```python
from build123d import *

# Parameters (mm, degrees)
SKIZZE1_W                        = 199
SKIZZE1_H                        = 420
AUFSATZ_LINEAR_AUSTRAGEN1_DEPTH  = 10
SKIZZE5_W                        = 199
SKIZZE5_H                        = 85
SCHNITT_LINEAR_AUSTRAGEN2_DEPTH  = 10
SKIZZE20_R                       = 1.7
SCHNITT_LINEAR_AUSTRAGEN12_DEPTH = 233.594604409
SKIZZE21_W                       = 134.422077922
SKIZZE21_H                       = 75
SCHNITT_LINEAR_AUSTRAGEN13_DEPTH = 233.594604409
SCHNITT_LINEAR_AUSTRAGEN14_DEPTH = 233.594604409
AUFSATZ_LINEAR_AUSTRAGEN6_DEPTH  = 10
SKIZZE25_R                       = 1.7
SCHNITT_LINEAR_AUSTRAGEN15_DEPTH = 233.594604409
SCHNITT_LINEAR_AUSTRAGEN16_DEPTH = 290.484023739
VERRUNDUNG1_R                    = 3
SKIZZE27_R                       = 1.7
SCHNITT_LINEAR_AUSTRAGEN17_DEPTH = 233.594604409
SCHNITT_LINEAR_AUSTRAGEN18_DEPTH = 5


with BuildPart() as part:
    # Skizze1 → Aufsatz-Linear austragen1 (new body)
    with BuildSketch(Plane(origin=(0, 0, 0), x_dir=(1, 0, 0), z_dir=(0, 1, 0))):
        Rectangle(SKIZZE1_W, SKIZZE1_H)
    extrude(amount=AUFSATZ_LINEAR_AUSTRAGEN1_DEPTH)

    # Skizze5 → Schnitt-Linear austragen2 (cut)
    with BuildSketch(Plane(origin=(0, 10, 0), x_dir=(1, 0, 0), z_dir=(0, 1, 0))):
        Polygon((99.5, -210), (18, -210), (99.5, -56), align=None)
        Polygon((-18, -210), (-99.5, -56), (-99.5, -210), align=None)
        with Locations((0, 167.5)):
            Rectangle(SKIZZE5_W, SKIZZE5_H)
        Polygon((67.211038961, -56), (-67.211038961, -56), (-2.646103896, -178), (2.646103896, -178), align=None)
    extrude(amount=-SCHNITT_LINEAR_AUSTRAGEN2_DEPTH, mode=Mode.SUBTRACT)

    # Skizze20 → Schnitt-Linear austragen12 (cut, through all)
    with BuildSketch(Plane(origin=(0, 10, 0), x_dir=(1, 0, 0), z_dir=(0, 1, 0))):
        with Locations(Location((90.5, 119.52, 0), (0, 0, 270))):
            Circle(SKIZZE20_R)
        with Locations(Location((48.5, 119.52, 0), (0, 0, 270))):
            Circle(SKIZZE20_R)
        with Locations(Location((-48.5, 119.52, 0), (0, 0, 90))):
            Circle(SKIZZE20_R)
        with Locations(Location((-90.5, 119.52, 0), (0, 0, 90))):
            Circle(SKIZZE20_R)
        with Locations(Location((87, 43.82, 0), (0, 0, 270))):
            Circle(SKIZZE20_R)
        with Locations(Location((52, 43.82, 0), (0, 0, 270))):
            Circle(SKIZZE20_R)
        with Locations(Location((-87, 43.82, 0), (0, 0, 90))):
            Circle(SKIZZE20_R)
        with Locations(Location((-52, 43.82, 0), (0, 0, 90))):
            Circle(SKIZZE20_R)
    extrude(amount=-SCHNITT_LINEAR_AUSTRAGEN12_DEPTH, mode=Mode.SUBTRACT)

    # Skizze21 → Schnitt-Linear austragen13 (cut, through all)
    with BuildSketch(Plane(origin=(0, 10, 0), x_dir=(1, 0, 0), z_dir=(0, 1, 0))):
        with Locations((0, -18.5)):
            Rectangle(SKIZZE21_W, SKIZZE21_H)
    extrude(amount=-SCHNITT_LINEAR_AUSTRAGEN13_DEPTH, mode=Mode.SUBTRACT)

    # Skizze22 → Schnitt-Linear austragen14 (cut, through all)
    with BuildSketch(Plane(origin=(0, 10, 0), x_dir=(1, 0, 0), z_dir=(0, 1, 0))):
        with BuildLine():
            Line((-67.211038961, -56), (-2.646103896, -178))
            ThreePointArc((-2.646103896, -178), (-52.825886854, -126.471631215), (-67.211038961, -56))
        make_face()
    schnitt_linear_austragen14 = extrude(amount=-SCHNITT_LINEAR_AUSTRAGEN14_DEPTH, mode=Mode.SUBTRACT)

    # Skizze23 → Aufsatz-Linear austragen6 (add)
    with BuildSketch(Plane(origin=(0, 10, 0), x_dir=(1, 0, 0), z_dir=(0, 1, 0))):
        with BuildLine():
            Line((-99.5, -56), (-18, -210))
            ThreePointArc((-18, -210), (-75.095260266, -141.650251374), (-99.5, -56))
        make_face()
    aufsatz_linear_austragen6 = extrude(amount=-AUFSATZ_LINEAR_AUSTRAGEN6_DEPTH)

    # Spiegeln2: Schnitt-Linear austragen14, Aufsatz-Linear austragen6 across plane
    add(schnitt_linear_austragen14.mirror(Plane(origin=(0, 0, 0), x_dir=(0, 0, 1), z_dir=(1, 0, 0))), mode=Mode.SUBTRACT)
    add(aufsatz_linear_austragen6.mirror(Plane(origin=(0, 0, 0), x_dir=(0, 0, 1), z_dir=(1, 0, 0))))

    # Skizze25 → Schnitt-Linear austragen15 (cut, through all)
    with BuildSketch(Plane(origin=(0, 10, 0), x_dir=(1, 0, 0), z_dir=(0, 1, 0))):
        with Locations(Location((-94.5, -11, 0), (0, 0, 270))):
            Circle(SKIZZE25_R)
        with Locations(Location((-72.211038961, -11, 0), (0, 0, 90))):
            Circle(SKIZZE25_R)
        with Locations(Location((-72.211038961, -51, 0), (0, 0, 270))):
            Circle(SKIZZE25_R)
        with Locations(Location((-94.5, -51, 0), (0, 0, 90))):
            Circle(SKIZZE25_R)
    schnitt_linear_austragen15 = extrude(amount=-SCHNITT_LINEAR_AUSTRAGEN15_DEPTH, mode=Mode.SUBTRACT)

    # Spiegeln3: Schnitt-Linear austragen15 across plane
    add(schnitt_linear_austragen15.mirror(Plane(origin=(0, 0, 0), x_dir=(0, 0, 1), z_dir=(1, 0, 0))), mode=Mode.SUBTRACT)

    # Skizze26 → Schnitt-Linear austragen16 (cut, through all)
    with BuildSketch(Plane.ZY.offset(99.5)):
        Polygon((56, 5), (56, 0), (4.196805737, -14.401746423), (-137.707729511, -14.401746423), (-137.707729511, 19.508660812), (5.012761814, 19.508660812), (6, 10), (6, 5), align=None)
    extrude(amount=-SCHNITT_LINEAR_AUSTRAGEN16_DEPTH, mode=Mode.SUBTRACT)

    # Verrundung1
    # the kernel refuses this fillet: 3 mm, written as the material it takes off along each edge
    with BuildSketch(Plane(origin=(60.076908998, 10, 66.721125619), x_dir=(-0.4390500946900349, 0, 0.8984625837243705), z_dir=(0.8984625837243705, 0, 0.4390500946900349))) as verrundung1_piece_1_section:
        with BuildLine():
            CenterArc((127.738655974 + VERRUNDUNG1_R, VERRUNDUNG1_R), VERRUNDUNG1_R, 180, 90)
            Line((127.738655974, VERRUNDUNG1_R), (127.738655974, 0))
            Line((127.738655974, 0), (127.738655974 + VERRUNDUNG1_R, 0))
        make_face()
    verrundung1_piece_1 = revolve(axis=Axis((60.076908998, 10, 66.721125619), (0, -1, 0)), revolution_arc=78.865488706, mode=Mode.PRIVATE)
    verrundung1_piece_1 = split(verrundung1_piece_1, bisect_by=Plane(origin=(60.076908998, 10, 178), z_dir=(0, 0, -1)), keep=Keep.TOP, mode=Mode.PRIVATE)
    add(verrundung1_piece_1, mode=Mode.SUBTRACT)
    with BuildSketch(Plane(origin=(-60.076908998, 10, 66.721125619), x_dir=(0.4390500946900349, 0, 0.8984625837243705), z_dir=(-0.8984625837243705, 0, 0.4390500946900349))) as verrundung1_piece_2_section:
        with BuildLine():
            CenterArc((127.738655974 + VERRUNDUNG1_R, -VERRUNDUNG1_R), VERRUNDUNG1_R, 90, 90)
            Line((127.738655974, -VERRUNDUNG1_R), (127.738655974, 0))
            Line((127.738655974, 0), (127.738655974 + VERRUNDUNG1_R, 0))
        make_face()
    verrundung1_piece_2 = revolve(axis=Axis((-60.076908998, 10, 66.721125619), (0, 1, 0)), revolution_arc=78.865488706, mode=Mode.PRIVATE)
    verrundung1_piece_2 = split(verrundung1_piece_2, bisect_by=Plane(origin=(-60.076908998, 10, 178), z_dir=(0, 0, -1)), keep=Keep.TOP, mode=Mode.PRIVATE)
    add(verrundung1_piece_2, mode=Mode.SUBTRACT)
    with BuildSketch(Plane(origin=(-10.146103896, 10, 178), x_dir=(0, 0, 1), z_dir=(1, 0, 0))) as verrundung1_piece_3_section:
        with BuildLine():
            CenterArc((VERRUNDUNG1_R, VERRUNDUNG1_R), VERRUNDUNG1_R, 180, 90)
            Line((0, VERRUNDUNG1_R), (0, 0))
            Line((0, 0), (VERRUNDUNG1_R, 0))
        make_face()
    verrundung1_piece_3 = extrude(amount=20.292207792, mode=Mode.PRIVATE)
    verrundung1_piece_3 = verrundung1_piece_3 & Plane(origin=(60.076908998, 10, 66.721125619), x_dir=(-0.4910260908528423, 0, 0.8711448663120137), z_dir=(0, 1, 0)) * Cylinder(127.738655974, 53, mode=Mode.PRIVATE)
    verrundung1_piece_3 = verrundung1_piece_3 & Plane(origin=(-60.076908998, 10, 66.721125619), x_dir=(0.4910260908528423, 0, 0.8711448663120137), z_dir=(0, 1, 0)) * Cylinder(127.738655974, 53, mode=Mode.PRIVATE)
    add(verrundung1_piece_3, mode=Mode.SUBTRACT)
    with BuildSketch(Plane(origin=(-10.146103896, 10, 178), x_dir=(0, 0, 1), z_dir=(1, 0, 0))) as verrundung1_piece_4_section:
        with BuildLine():
            CenterArc((VERRUNDUNG1_R, VERRUNDUNG1_R), VERRUNDUNG1_R, 180, 90)
            Line((0, VERRUNDUNG1_R), (0, 0))
            Line((0, 0), (VERRUNDUNG1_R, 0))
        make_face()
    verrundung1_piece_4 = extrude(amount=20.292207792, mode=Mode.PRIVATE)
    verrundung1_piece_4 = verrundung1_piece_4 - Plane(origin=(60.076908998, 10, 66.721125619), x_dir=(-0.4910260908528423, 0, 0.8711448663120137), z_dir=(0, 1, 0)) * Cylinder(127.738655974, 53, mode=Mode.PRIVATE)
    verrundung1_piece_4 = verrundung1_piece_4 - Plane(origin=(-60.076908998, 10, 66.721125619), x_dir=(0.4910260908528423, 0, 0.8711448663120137), z_dir=(0, 1, 0)) * Cylinder(127.738655974, 53, mode=Mode.PRIVATE)
    add(verrundung1_piece_4, mode=Mode.SUBTRACT)
    with BuildSketch(Plane(origin=(60.076908998, 10, 66.721125619), x_dir=(-0.4390500946900349, 0, 0.8984625837243705), z_dir=(0.8984625837243705, 0, 0.4390500946900349))) as verrundung1_piece_5a_section:
        with BuildLine():
            CenterArc((127.738655974 + VERRUNDUNG1_R, VERRUNDUNG1_R), VERRUNDUNG1_R, 180, 90)
            Line((127.738655974, VERRUNDUNG1_R), (127.738655974, 0))
            Line((127.738655974, 0), (127.738655974 + VERRUNDUNG1_R, 0))
        make_face()
    verrundung1_piece_5a = revolve(axis=Axis((60.076908998, 10, 66.721125619), (0, -1, 0)), revolution_arc=78.865488706, mode=Mode.PRIVATE)
    verrundung1_piece_5a = split(verrundung1_piece_5a, bisect_by=Plane(origin=(60.076908998, 10, 178), z_dir=(0, 0, 1)), keep=Keep.TOP, mode=Mode.PRIVATE)
    with BuildSketch(Plane(origin=(-10.146103896, 10, 178), x_dir=(0, 0, 1), z_dir=(1, 0, 0))) as verrundung1_piece_5b_section:
        with BuildLine():
            CenterArc((VERRUNDUNG1_R, VERRUNDUNG1_R), VERRUNDUNG1_R, 180, 90)
            Line((0, VERRUNDUNG1_R), (0, 0))
            Line((0, 0), (VERRUNDUNG1_R, 0))
        make_face()
    verrundung1_piece_5b = extrude(amount=20.292207792, mode=Mode.PRIVATE)
    verrundung1_piece_5b = verrundung1_piece_5b - Plane(origin=(60.076908998, 10, 66.721125619), x_dir=(-0.4910260908528423, 0, 0.8711448663120137), z_dir=(0, 1, 0)) * Cylinder(127.738655974, 53, mode=Mode.PRIVATE)
    verrundung1_piece_5b = verrundung1_piece_5b & Plane(origin=(-60.076908998, 10, 66.721125619), x_dir=(0.4910260908528423, 0, 0.8711448663120137), z_dir=(0, 1, 0)) * Cylinder(127.738655974, 53, mode=Mode.PRIVATE)
    verrundung1_piece_5 = verrundung1_piece_5a & verrundung1_piece_5b
    add(verrundung1_piece_5, mode=Mode.SUBTRACT)
    with BuildSketch(Plane(origin=(-10.146103896, 10, 178), x_dir=(0, 0, 1), z_dir=(1, 0, 0))) as verrundung1_piece_6a_section:
        with BuildLine():
            CenterArc((VERRUNDUNG1_R, VERRUNDUNG1_R), VERRUNDUNG1_R, 180, 90)
            Line((0, VERRUNDUNG1_R), (0, 0))
            Line((0, 0), (VERRUNDUNG1_R, 0))
        make_face()
    verrundung1_piece_6a = extrude(amount=20.292207792, mode=Mode.PRIVATE)
    verrundung1_piece_6a = verrundung1_piece_6a & Plane(origin=(60.076908998, 10, 66.721125619), x_dir=(-0.4910260908528423, 0, 0.8711448663120137), z_dir=(0, 1, 0)) * Cylinder(127.738655974, 53, mode=Mode.PRIVATE)
    verrundung1_piece_6a = verrundung1_piece_6a - Plane(origin=(-60.076908998, 10, 66.721125619), x_dir=(0.4910260908528423, 0, 0.8711448663120137), z_dir=(0, 1, 0)) * Cylinder(127.738655974, 53, mode=Mode.PRIVATE)
    with BuildSketch(Plane(origin=(-60.076908998, 10, 66.721125619), x_dir=(0.4390500946900349, 0, 0.8984625837243705), z_dir=(-0.8984625837243705, 0, 0.4390500946900349))) as verrundung1_piece_6b_section:
        with BuildLine():
            CenterArc((127.738655974 + VERRUNDUNG1_R, -VERRUNDUNG1_R), VERRUNDUNG1_R, 90, 90)
            Line((127.738655974, -VERRUNDUNG1_R), (127.738655974, 0))
            Line((127.738655974, 0), (127.738655974 + VERRUNDUNG1_R, 0))
        make_face()
    verrundung1_piece_6b = revolve(axis=Axis((-60.076908998, 10, 66.721125619), (0, 1, 0)), revolution_arc=78.865488706, mode=Mode.PRIVATE)
    verrundung1_piece_6b = split(verrundung1_piece_6b, bisect_by=Plane(origin=(-60.076908998, 10, 178), z_dir=(0, 0, 1)), keep=Keep.TOP, mode=Mode.PRIVATE)
    verrundung1_piece_6 = verrundung1_piece_6a & verrundung1_piece_6b
    add(verrundung1_piece_6, mode=Mode.SUBTRACT)

    # Skizze27 → Schnitt-Linear austragen17 (cut, through all)
    with BuildSketch(Plane(origin=(0, 10, 0), x_dir=(1, 0, 0), z_dir=(0, 1, 0))):
        with Locations(Location((28.5, -179.171533214, 0), (0, 0, 270))):
            Circle(SKIZZE27_R)
        with Locations(Location((21.5, -201.421972318, 0), (0, 0, 270))):
            Circle(SKIZZE27_R)
        with Locations(Location((-21.5, -201.421972318, 0), (0, 0, 90))):
            Circle(SKIZZE27_R)
        with Locations(Location((-28.5, -179.171533214, 0), (0, 0, 90))):
            Circle(SKIZZE27_R)
    extrude(amount=-SCHNITT_LINEAR_AUSTRAGEN17_DEPTH, mode=Mode.SUBTRACT)

    # Skizze28 → Schnitt-Linear austragen18 (cut)
    with BuildSketch(Plane.XZ):
        Polygon((21.5, 204.828338906), (24.45, 203.125155612), (24.45, 199.718789024), (21.5, 198.01560573), (18.55, 199.718789024), (18.55, 203.125155612), align=None)
        Polygon((28.5, 182.577899803), (31.45, 180.874716508), (31.45, 177.46834992), (28.5, 175.765166626), (25.55, 177.46834992), (25.55, 180.874716508), align=None)
        Polygon((-28.5, 182.577899803), (-25.55, 180.874716508), (-25.55, 177.46834992), (-28.5, 175.765166626), (-31.45, 177.46834992), (-31.45, 180.874716508), align=None)
        Polygon((-21.5, 204.828338906), (-18.55, 203.125155612), (-18.55, 199.718789024), (-21.5, 198.01560573), (-24.45, 199.718789024), (-24.45, 203.125155612), align=None)
    extrude(amount=-SCHNITT_LINEAR_AUSTRAGEN18_DEPTH, mode=Mode.SUBTRACT)


solid = part.part
```
For this review, take the finished solid that the model builds, in its own axes (mm). A direction names the side the tool comes from. Coordinates: 2 decimals unless noted, no trailing zeros. Write each loop counter-clockwise with the first axis right and the second up, starting at its lowest first coordinate (ties: lowest second). Pieces come first, ordered by that corner, then holes.
(1) The part is to be moulded in two halves that separate along Z. For faces 5 (the face through (-74.505, 5.07, 142.759)), 6 (the face through (23, 5, 200)), 7 (the face through (-99.5, 7, 31)), say which applies: +Z half, -Z half, draft (parallel to the pull), parting line (faces both ways), or undercut.
(2) Wall thickness on probe 1 along X at (y, z) = (8.9, 11); probe 2 along Y at (x, z) = (76.5, 35.5); probe 3 along X at (y, z) = (8, 125.5): over which ranges is each line inside the solid? List them lowest first.
(3) Add section A-A on z = 29. Give the boundary of the cut face in (x, y), then the cut area to 3 significant figures.
(4) Add section B-B on y = 2. Count the separate pieces of the cut face and the enclosed holes in it, then the cut area to 4 significant figures.
(5) Tool access review of faces 1 (the face through (0, 4, 178)), 2 (the face through (-84, 3, 56)), 3 (the face through (30, 5, 178)), 4 (the face through (83, 8, 6)): name each direction out of +Z, -Z, +X, -X, +Y, -Y from which nothing blocks a thin tool from reaching the whole face with its end or side.
(6) For pin 1 Ø1.7 at (y, z) = (1.5, 178.5) entering from -X; pin 2 Ø6 at (y, z) = (5.5, 92) entering from -X; pin 3 Ø3.5 at (y, z) = (1.5, 179.5) entering from -X; pin 4 Ø2 at (x, z) = (72.21, 51) entering from +Y, all flat-tipped, find the tip position at first contact; note any pin that passes through.
Answer sheet:
1. face 5: +Z half
1. face 6: undercut
1. face 7: draft
2. probe 1: x = -99.5 to -96.2, -92.8 to -73.91, -70.51 to -67.21, 67.21 to 70.51, 73.91 to 92.8, 96.2 to 99.5
2. probe 2: y = 5 to 10
2. probe 3: x = -82.8 to -53.53, 53.53 to 82.8
3. outline: (-99.5, 5) - (-67.21, 5) - (-67.21, 10) - (-99.5, 10) - close; (67.21, 5) - (99.5, 5) - (99.5, 10) - (67.21, 10) - close
3. area: 323 mm2
4. separate pieces: 1
4. enclosed holes: 4
4. area: 10,000 mm2
5. face 1: -Z, +Y, -Y
5. face 2: -Z, +X, -X, -Y
5. face 3: -Y
5. face 4: -Z, +X, -X, +Y, -Y
6. pin 1: stops at x = -51.11
6. pin 2: stops at x = -94.64
6. pin 3: stops at x = -51.02
6. pin 4: passes through
